```python
from build123d import *

# Parameters (mm, degrees)
BOSS_EXTRUDE1_DEPTH = 5
FILLET1_R           = 2.5
FILLET2_R           = 5


with BuildPart() as part:
    # Sketch1 → Boss-Extrude1 (new body)
    with BuildSketch(Plane(origin=(0, 0, 0), x_dir=(1, 0, 0), z_dir=(0, 1, 0))):
        with BuildLine():
            ThreePointArc((11.980797937, 135.715861366), (0, 124.394448725), (-11.980797937, 135.715861366))
            ThreePointArc((-11.980797937, 135.715861366), (-10.495298574, 100.729871278), (-10, 65.715861366))
            Line((-10, 65.715861366), (-10, 0))
            ThreePointArc((-10, 0), (0, -10), (10, 0))
            Line((10, 0), (10, 65.715861366))
            ThreePointArc((10, 65.715861366), (10.495298574, 100.729871278), (11.980797937, 135.715861366))
        make_face()
        with BuildLine():
            Line((-6, 140), (-7.957050212, 145.376951267))
            ThreePointArc((-7.957050212, 145.376951267), (0, 124.394448725), (7.957050212, 145.376951267))
            Line((7.957050212, 145.376951267), (6, 140))
            ThreePointArc((6, 140), (0, 129.394448725), (-6, 140))
        make_face()
    extrude(amount=BOSS_EXTRUDE1_DEPTH)

    # Fillet1
    fillet1_edges = [part.edges().sort_by_distance(p)[0] for p in [
        (11.077617601, 0, -141.008166128),
        (10.495298574, 0, -100.729871278),
        (10, 0, -32.857930683),
        (0, 0, 10),
        (-10, 0, -32.857930683),
        (-10.495298574, 0, -100.729871278),
        (11.077617601, 5, -141.008166128),
        (10.495298574, 5, -100.729871278),
        (10, 5, -32.857930683),
        (0, 5, 10),
        (-10, 5, -32.857930683),
        (-10.495298574, 5, -100.729871278),
        (-11.077617601, 0, -141.008166128),
        (-11.077617601, 5, -141.008166128),
    ]]
    fillet(fillet1_edges, radius=FILLET1_R - 0.0001)  # a hair under: the kernel refuses the full size

    # Fillet2
    fillet2_edges = [part.edges().sort_by_distance(p)[0] for p in [
        (-6, 2.5, -140),
        (6, 2.5, -140),
    ]]
    fillet(fillet2_edges, radius=FILLET2_R)


solid = part.part
```
Can you work these out from the model? Positions are in its coordinate system, mm. A direction names the side the tool comes from. Give positions to 0.01 mm unless a question says otherwise; leave off trailing zeros. Loops run counter-clockwise (first coordinate to the right, second up) from the corner with the lowest first, then second, coordinate; pieces in that order, holes last. Notation, with made-up numbers: M 13,88 L 66,88 A20 cw 66,100 Z; hole C 44.25,-34.75 d3. An arc over 180 degrees is marked long. One line per item, written item: value.
(1) I need wall thicknesses on line 1 (Z direction, x = 0, y = 2.45); line 2 (Y direction, x = 8.25, z = -100); line 3 (X direction, y = 2.7, z = -86). Which ranges of each line are inside material? Lowest first, please.
Returned:
line 1: -129.39 to 10
line 2: 0.02 to 4.98
line 3: -10.16 to 10.16
(2) We'd pull the mould along X, two halves only. Please class faces 1 (the face through (-6.388, 2.535, -140.275)), 2 (the face through (0, 0, -69)), 3 (the face through (9.287, 4.248, -33.318)), 4 (the face through (-9.287, 4.248, -32.398)): released by +X, released by -X, zero draft, split by the parting line, or undercut.
Returned:
face 1: undercut
face 2: zero draft
face 3: released by +X
face 4: released by -X
(3) Which directions (+Z, -Z, +X, -X, +Y, -Y) give clear straight access to the entire face, cutting with the end or side of a thin tool? Please do faces 5 (the face through (-9.287, 0.752, -32.398)), 6 (the face through (9.287, 0.752, -33.318)), 7 (the face through (6.387, 2.535, -140.228)), 8 (the face through (7.2, 2.5, -143.3)), 9 (the face through (0, 5, -69)).
Returned:
face 5: +Z, -X, -Y
face 6: +Z, +X, -Y
face 7: +Y, -Y
face 8: -Z, +Y, -Y
face 9: +Z, -Z, +X, -X, +Y
(4) Will these pins go through, and if not, where does the flat tip stop? pin 1 (1.5 mm diameter, centred on x = 7.5, y = 3.5, fed in from -Z) (3 decimals); pin 2 (1.5 mm diameter, centred on y = 2, z = -35, fed in from -X).
Returned:
pin 1: z = -145.345
pin 2: x = -10
(5) Suppose I cut it at C-C on y = 0.85. List the corners of the cut face in (x, z) for me.
Returned:
outline: M -11.36,-135.75 A11.38 ccw -7.73,-144.75 L -6.69,-141.89 A5 ccw -6.64,-138.6 A7 cw long 6.64,-138.6 A5 ccw 6.69,-141.89 L 7.73,-144.75 A11.38 ccw 11.36,-135.75 A1238.49 cw 9.38,-65.72 L 9.38,0 A9.38 ccw -9.38,0 L -9.38,-65.72 A1238.49 cw Z
